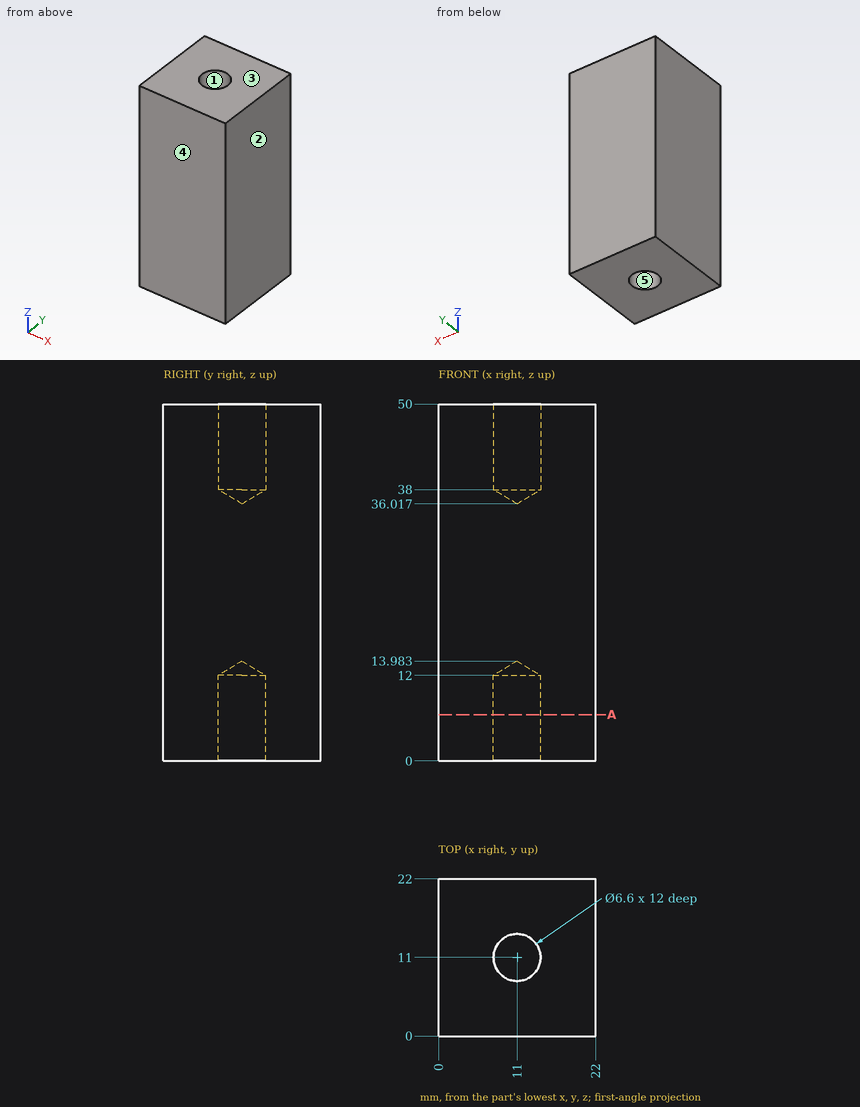
Study the drawing (mm; zero at the part's minimum x, y, z) and answer. A direction names the side the tool comes from. Give positions to 0.01 mm unless a question says otherwise; leave off trailing zeros. Order: outer loops, then holes, each group sorted by start corner. A loop starts at its lowest first (then second) coordinate and runs counter-clockwise, first axis right, second up. Notation, with made-up numbers: M -29.75,3 L -2.75,3 A32 cw -2.75,34 Z; hole C 51,22.25 d6. An arc over 180 degrees is marked long. Put each result on its own line as item: value. Start each with the question number.
Item 1: For a pull along X with two mould halves and no side action, classify the marked faces 1, 2 and 3 as +X half, -X half, draft (parallel to the pull), parting line (faces both ways), or undercut.
Item 2: The part is cut by section A-A, the plane z = 6.5. Determine the outline of the cut face in (x, y), and give its area (3 significant figures).
Item 3: A flat-ended cylindrical pin translates along its axis: P1, Ø3, axis at x = 10.5, y = 10, coming from the +Z side. Find the tip coordinate at first contact, or state that the pin passes through.
Item 4: Which of the six approach directions +Z, -Z, +X, -X, +Y, -Y give full straight-line access (tool end or side, diameter ignored) to the marked faces 4 and 5?
Item 5: Find the intervals of material crossed by line 1 along Y through (x, z) = (11, 42.5); line 2 along Z through (x, y) = (12.5, 11.75) (1 decimal), in increasing order.
Answer key:
1. face 1: undercut
1. face 2: +X half
1. face 3: draft
2. outline: M 0,0 L 22,0 L 22,22 L 0,22 Z; hole C 11,11 d6.6
2. area: 450 mm²
3. P1: stops at z = 37.59
4. face 4: +Z, -Z, +X, -X, -Y
4. face 5: -Z
5. line 1: y = 0 to 7.7, 14.3 to 22
5. line 2: z = 13 to 37
